The model under review builds one solid part; all positions refer to its coordinate system, in mm. Face numbers are marked on the shaded views. A direction names the side the tool comes from. Round coordinates to 2 decimals unless told otherwise and drop trailing zeros. Loops run counter-clockwise (first coordinate to the right, second up) from the corner with the lowest first, then second, coordinate; pieces in that order, holes last. Notation, with made-up numbers: M 3.5,41.5 L 56.5,41.5 A8 cw 56.5,53.5 Z; hole C 11,56.5 d9. An arc over 180 degrees is marked long. One line per question, with ' | ' between items.
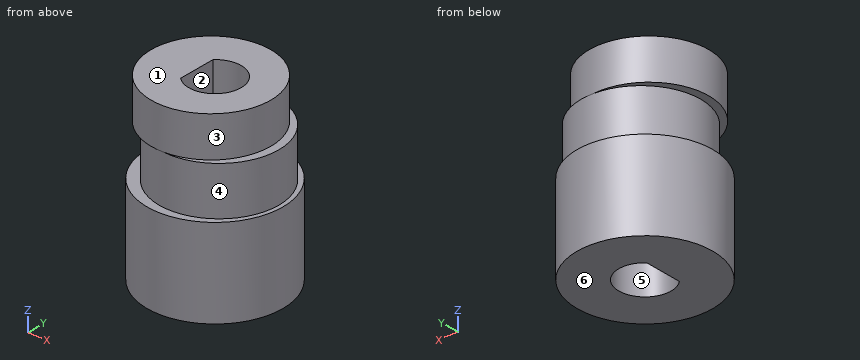
from build123d import *

# Parameters (mm, degrees)
ESQUISSE1_R             = 8.4
BOSS_EXTRU_1_DEPTH      = 11
ESQUISSE3_R             = 7.4
BOSS_EXTRU_2_DEPTH      = 6
ESQUISSE4_R             = 7.4
BOSS_EXTRU_3_DEPTH      = 5
ENL_V_MAT_EXTRU_1_DEPTH = 26.002399885


with BuildPart() as part:
    # Esquisse1 → Boss.-Extru.1 (new body)
    with BuildSketch(Plane.XY):
        Circle(ESQUISSE1_R)
    extrude(amount=BOSS_EXTRU_1_DEPTH)

    # Esquisse3 → Boss.-Extru.2 (add)
    with BuildSketch(Plane.XY.offset(11)):
        with Locations((0.5, 0)):
            Circle(ESQUISSE3_R)
    extrude(amount=BOSS_EXTRU_2_DEPTH)

    # Esquisse4 → Boss.-Extru.3 (add)
    with BuildSketch(Plane.XY.offset(17)):
        with Locations(Location((-0.5, 0, 0), (0, 0, 273.874288206))):
            Circle(ESQUISSE4_R)
    extrude(amount=BOSS_EXTRU_3_DEPTH)

    # Esquisse5 → Enlèv. mat.-Extru.1 (cut, through all)
    with BuildSketch(Plane(origin=(0, 0, 0), x_dir=(-1, 0, 0), z_dir=(0, 0, -1))):
        with BuildLine():
            Line((2.25, 2.34520788), (2.25, -2.34520788))
            ThreePointArc((2.25, -2.34520788), (-3.25, 0), (2.25, 2.34520788))
        make_face()
    extrude(amount=-ENL_V_MAT_EXTRU_1_DEPTH, mode=Mode.SUBTRACT)


solid = part.part
1) Add section B-B on x = -0.5. State the section outline as (y, z) points, then the cut area to 3 significant figures.
Output values:
outline: M -8.39,0 L -3.21,0 L -3.21,22 L -7.4,22 L -7.4,17 L -7.33,17 L -7.33,11 L -8.39,11 Z; M 3.21,0 L 8.39,0 L 8.39,11 L 7.33,11 L 7.33,17 L 7.4,17 L 7.4,22 L 3.21,22 Z | area: 205 mm²
2) Insertion check: P1, Ø10, axis at x = 0, z = 18.5, coming from the -Y side; P2, Ø1, axis at x = -5, z = 7, coming from the +Y side; P3, Ø6, axis at y = 1, z = 15, coming from the -X side. Each pin has a flat end and moves straight along its axis. Give the tip position at first contact, or say it passes through.
Output values:
P1: stops at y = -7.4 | P2: stops at y = 7.09 | P3: stops at x = -7.9
3) Add section C-C on z = 8.75. State the section outline as (x, y) points, then the cut area to 3 significant figures.
Output values:
outline: C 0,0 d16.8; hole M -2.25,-2.35 A3.25 ccw long -2.25,2.35 Z | area: 192 mm²
4) Machinability: for the marked faces 1, 2 and 3, which of the approach directions +Z, -Z, +X, -X, +Y, -Y give a long, thin tool a straight path to every point of the face, cutting with its end or side? Answer none if there is none.
Output values:
face 1: +Z, +X, -X, +Y, -Y | face 2: +Z, -Z | face 3: +Z
5) Mouldability with a two-part tool opening along Y and no side actions: class the marked faces 4, 5 and 6 as +Y half, -Y half, draft (parallel to the pull), parting line (faces both ways), or undercut.
Output values:
face 4: parting line | face 5: undercut | face 6: draft
6) Add section A-A on y = 0. State the section outline as (x, z) points, then the cut area to 3 significant figures.
Output values:
outline: M -8.4,0 L -2.25,0 L -2.25,22 L -7.9,22 L -7.9,17 L -6.9,17 L -6.9,11 L -8.4,11 Z; M 3.25,0 L 8.4,0 L 8.4,11 L 7.9,11 L 7.9,17 L 6.9,17 L 6.9,22 L 3.25,22 Z | area: 227 mm²
7) For line 1 (X direction, y = 0, z = 13.25); line 2 (Y direction, x = 0, z = 7.25); line 3 (Z direction, x = -7, y = -0.5), list the stretches that pass through material, from the lowest coordinate up.
Output values:
line 1: x = -6.9 to -2.25, 3.25 to 7.9 | line 2: y = -8.4 to -3.25, 3.25 to 8.4 | line 3: z = 0 to 11, 17 to 22
8) Add section D-D on x = 4.5. State the section outline as (y, z) points.
Output values:
outline: M -7.09,0 L 7.09,0 L 7.09,11 L 6.23,11 L 6.23,17 L 5.46,17 L 5.46,22 L -5.46,22 L -5.46,17 L -6.23,17 L -6.23,11 L -7.09,11 Z
